Verification items for the finished model (mm, model axes). Face numbers are marked on the shaded views. A direction names the side the tool comes from. Coordinates: 2 decimals unless noted, no trailing zeros. Order: outer loops, then holes, each group sorted by start corner. A loop starts at its lowest first (then second) coordinate and runs counter-clockwise, first axis right, second up. Notation, with made-up numbers: M 5,48 L 18,48 A27 cw 18,72 Z; hole C 86,-36 d3. An arc over 180 degrees is marked long. Return JSON: item names as keys, results as strings. Group by question number.
Q1. Section check D-D, the plane y = 2. Enter the section's corners in (x, z).
Q2. Go/stop test with flat-tipped pins: pin 1 Ø6 at (x, z) = (-7, 2.5) entering from -Y; pin 2 Ø3 at (x, z) = (-6.5, -1.5) entering from +Y; pin 3 Ø5 at (y, z) = (3.5, 8) entering from +X. Record where each tip stops, or that it passes through.
Q3. Thickness scan on probe 1 along X at (y, z) = (1.25, 0); probe 2 along Y at (x, z) = (1.25, -5.75); probe 3 along X at (y, z) = (3.75, -9.5). Record the ranges inside material, lowest first.
Q4. Section check A-A, the plane z = 0. Enter the section's corners in (x, y).
Q5. Section check B-B, the plane x = 0. Enter the section's corners in (y, z), then the cut area to 3 significant figures.
Q6. Access from +Z, -Z, +X, -X, +Y, -Y to the whole of each face (thin tool, end or side, straight path). Record for the marked faces 1 and 2.
Q7. Section check C-C, the plane y = 5.25. Enter the section's corners in (x, z).
Q8. Mould release check, pull along X, two halves, no side actions. Record for the marked faces 3, 4 and 5: pulls with the +X half, pulls with the -X half, needs draft (parallel to the pull), parting line crosses it, or undercut.
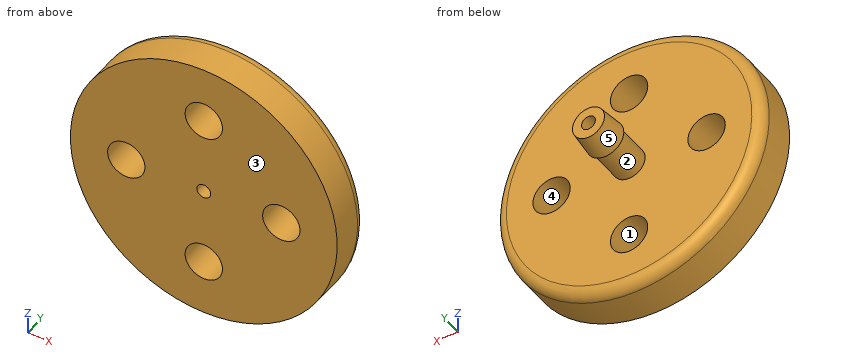
from build123d import *

# Parameters (mm, degrees)
SKETCH1_R           = 12.5
BOSS_EXTRUDE1_DEPTH = 4
SKETCH2_R           = 1.5
BOSS_EXTRUDE2_DEPTH = 6
FILLET1_R           = 1
CUT_EXTRUDE1_REACH  = 22.31
SKETCH6_R           = 0.65
CUT_EXTRUDE2_REACH  = 22.31
SKETCH7_R           = 1.75
CIRPATTERN1_COUNT   = 4


with BuildPart() as part:
    # Sketch1 → Boss-Extrude1 (new body)
    with BuildSketch(Plane(origin=(0, 0, 0), x_dir=(1, 0, 0), z_dir=(0, 1, 0))):
        with Locations(Location((0, 0, 0), (0, 0, 270))):
            Circle(SKETCH1_R)
    extrude(amount=BOSS_EXTRUDE1_DEPTH)

    # Sketch2 → Boss-Extrude2 (add)
    with BuildSketch(Plane(origin=(0, 4, 0), x_dir=(1, 0, 0), z_dir=(0, 1, 0))):
        with Locations(Location((0, 0, 0), (0, 0, 270))):
            Circle(SKETCH2_R)
    extrude(amount=BOSS_EXTRUDE2_DEPTH)

    # Fillet1
    fillet1_edges = [part.edges().sort_by_distance(p)[0] for p in [
        (0, 4, -12.5),
    ]]
    fillet(fillet1_edges, radius=FILLET1_R)

    # Sketch5 → Revolve1 (revolve)
    with BuildSketch(Plane.XY, mode=Mode.PRIVATE) as revolve1_sk:
        Polygon((0, 7.54), (0, 10), (1.5, 10), (1.75, 7.54), align=None)
    revolve(revolve1_sk.sketch.rotate(Axis((0, 7.54, 0), (0, 1, 0)), 90), axis=Axis((0, 7.54, 0), (0, 1, 0)))

    # Sketch6 → Cut-Extrude1 (cut, up to next)
    with BuildSketch(Plane.XZ, mode=Mode.PRIVATE) as cut_extrude1_sk1:
        with Locations(Location((0, 0, 0), (0, 0, 270))):
            Circle(SKETCH6_R)
    cut_extrude1_tool1 = extrude(cut_extrude1_sk1.sketch, amount=-CUT_EXTRUDE1_REACH, mode=Mode.PRIVATE) & part.part
    add(cut_extrude1_tool1.solids().sort_by_distance((0, 0, 0))[0], mode=Mode.SUBTRACT)

    # Sketch7 → Cut-Extrude2 (cut, up to next)
    with BuildSketch(Plane.XZ, mode=Mode.PRIVATE) as cut_extrude2_sk1:
        with Locations(Location((-7.263210785, 0, 0), (0, 0, 270))):
            Circle(SKETCH7_R)
    cut_extrude2_tool1 = extrude(cut_extrude2_sk1.sketch, amount=-CUT_EXTRUDE2_REACH, mode=Mode.PRIVATE) & part.part
    cut_extrude2 = cut_extrude2_tool1.solids().sort_by_distance((-7.263211, 0, 0))[0]
    add(cut_extrude2, mode=Mode.SUBTRACT)

    # CirPattern1: Cut-Extrude2 ×4 about axis
    cirpattern1_axis = Axis((0, 0, 0), (0, 1, 0))
    for i in range(1, CIRPATTERN1_COUNT):
        add(cut_extrude2.rotate(cirpattern1_axis, i * 360 / CIRPATTERN1_COUNT), mode=Mode.SUBTRACT)


solid = part.part
Numbers:
{
 "1": {"outline": "C 0,0 d25; hole C -7.26,0 d3.5; hole C 0,-7.26 d3.5; hole C 0,7.26 d3.5; hole C 0,0 d1.3; hole C 7.26,0 d3.5"},
 "2": {"pin 1": "stops at y = 0", "pin 2": "stops at y = 4", "pin 3": "stops at x = 11.2"},
 "3": {"probe 1": "x = -12.5 to -9.01, -5.51 to -0.65, 0.65 to 5.51, 9.01 to 12.5", "probe 2": "y = 0 to 4", "probe 3": "x = -7.59 to 7.59"},
 "4": {"outline": "M -12.5,0 L -9.01,0 L -9.01,4 L -11.5,4 A1 ccw -12.5,3 Z; M -5.51,0 L -0.65,0 L -0.65,10 L -1.5,10 L -1.75,7.54 L -1.5,7.54 L -1.5,4 L -5.51,4 Z; M 0.65,0 L 5.51,0 L 5.51,4 L 1.5,4 L 1.5,7.54 L 1.75,7.54 L 1.5,10 L 0.65,10 Z; M 9.01,0 L 12.5,0 L 12.5,3 A1 ccw 11.5,4 L 9.01,4 Z"},
 "5": {"outline": "M 0,-12.5 L 3,-12.5 A1 ccw 4,-11.5 L 4,-9.01 L 0,-9.01 Z; M 0,-5.51 L 4,-5.51 L 4,-1.5 L 7.54,-1.5 L 7.54,-1.75 L 10,-1.5 L 10,-0.65 L 0,-0.65 Z; M 0,0.65 L 10,0.65 L 10,1.5 L 7.54,1.75 L 7.54,1.5 L 4,1.5 L 4,5.51 L 0,5.51 Z; M 0,9.01 L 4,9.01 L 4,11.5 A1 ccw 3,12.5 L 0,12.5 Z", "area": "77.2 mm2"},
 "6": {"face 1": "+Y, -Y", "face 2": "none"},
 "7": {"outline": "C 0,0 d3; hole C 0,0 d1.3"},
 "8": {"face 3": "needs draft", "face 4": "undercut", "face 5": "parting line crosses it"}
}
